Verification items for this drawing (mm, ordinates from the low corner). A direction names the side the tool comes from. Coordinates: 2 decimals unless noted, no trailing zeros. Write each loop counter-clockwise with the first axis right and the second up, starting at its lowest first coordinate (ties: lowest second). Pieces come first, ordered by that corner, then holes. Notation, with made-up numbers: (43, -17) -> (90, -17) arc R15 cw to (90, -7) -> close; hole circle Ø10 at (11, 50). An arc over 180 degrees is marked (long way). Put each result on its own line as item: value. Start each with the question number.
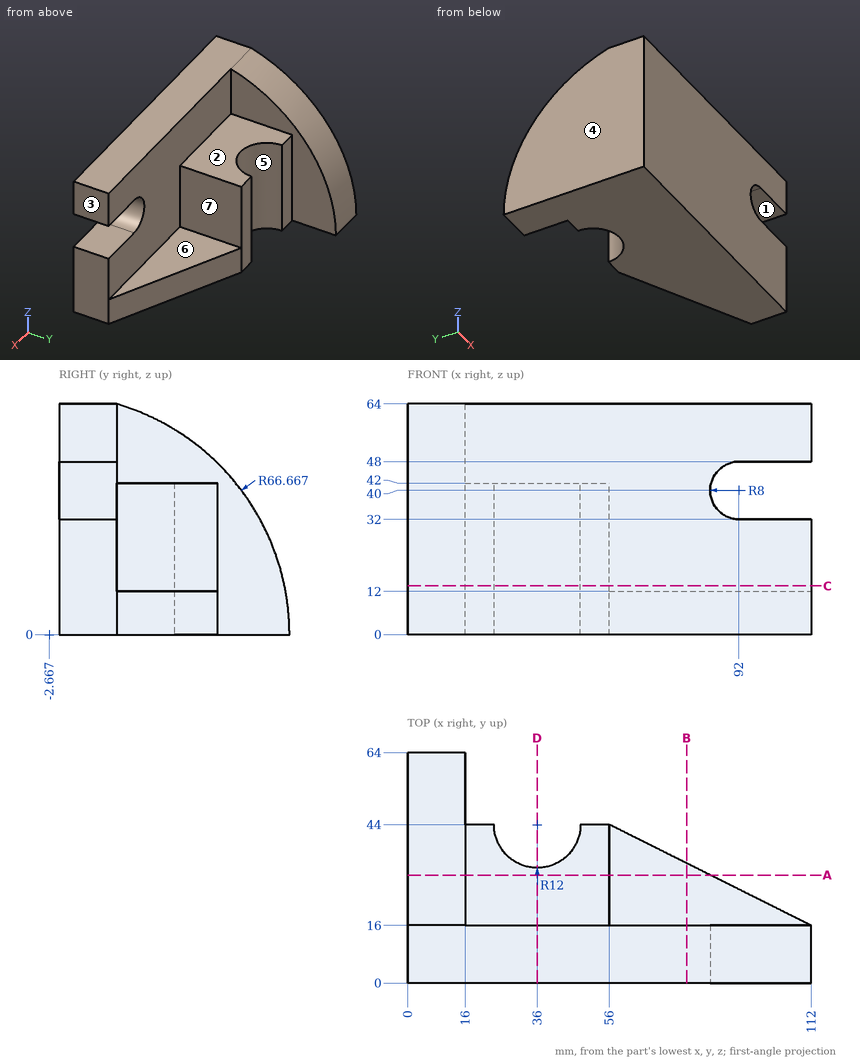
Item 1: Access from +Z, -Z, +X, -X, +Y, -Y to the whole of each face (thin tool, end or side, straight path). Record for the marked faces 1, 2 and 3.
Item 2: Section check B-B, the plane x = 77.5. Enter the section's corners in (y, z), and give its area (3 significant figures).
Item 3: Section check D-D, the plane x = 36. Enter the section's corners in (y, z), and give its area (3 significant figures).
Item 4: Section check A-A, the plane y = 30. Enter the section's corners in (x, z) (1 decimal), and give its area (3 significant figures).
Item 5: Mould release check, pull along X, two halves, no side actions. Record for the marked faces 4, 5, 6 and 7: released by +X, released by -X, zero draft, split by the parting line, or undercut.
Item 6: Scan lines: line 1 along X through (y, z) = (35.5, 46.5); line 2 along X through (y, z) = (20.5, 18.5). Record each from-to range of solid material in increasing order. Write a range as [from, to].
Item 7: Section check C-C, the plane z = 13.5. Enter the section's corners in (x, y), and give its area (3 significant figures).
Item 8: Go/stop test with flat-tipped pins: P1, Ø2.5, axis at x = 19.5, z = 13, coming from the +Y side; P2, Ø2, axis at x = 34.5, y = 28.5, coming from the -Z side; P3, Ø8, axis at y = 53.5, z = 12, coming from the +X side; P4, Ø22.5, axis at x = 96.5, y = 36, coming from the +Z side. Record where each tip stops, or that it passes through.
From the geometry:
1. face 1: +X, +Y, -Y
1. face 2: +Z, +X, +Y
1. face 3: +Z, -Z, +X, +Y, -Y
2. outline: (0, 0) -> (33.25, 0) -> (33.25, 12) -> (16, 12) -> (16, 64) -> (0, 64) -> close
2. area: 1,230 mm²
3. outline: (0, 0) -> (32, 0) -> (32, 42) -> (16, 42) -> (16, 64) -> (0, 64) -> close
3. area: 1,700 mm²
4. outline: (0, 0) -> (84, 0) -> (84, 12) -> (56, 12) -> (56, 42) -> (16, 42) -> (16, 58.1) -> (0, 58.1) -> close
4. area: 2,950 mm²
5. face 4: released by -X
5. face 5: undercut
5. face 6: zero draft
5. face 7: released by +X
6. line 1: [0, 16]
6. line 2: [0, 56]
7. outline: (0, 0) -> (112, 0) -> (112, 16) -> (56, 16) -> (56, 44) -> (48, 44) arc R12 cw to (24, 44) -> (16, 44) -> (16, 62.62) -> (0, 62.62) -> close
7. area: 3,430 mm²
8. P1: y = 44
8. P2: z = 0
8. P3: x = 16
8. P4: z = 12
